Check sheet for the modelled part. Datum: model origin and axes. Units: mm. A direction names the side the tool comes from. Round coordinates to 2 decimals unless told otherwise and drop trailing zeros. Order: outer loops, then holes, each group sorted by start corner. A loop starts at its lowest first (then second) coordinate and runs counter-clockwise, first axis right, second up.
(1) Sectioned sample at A-A, the plane z = -3. Enter the section's corners in (x, y) (3 decimals).
(2) Thickness scan on probe 1 along Y at (x, z) = (38, 56.5); probe 2 along Z at (x, y) = (-33.5, 32.5) (3 decimals); probe 3 along Y at (x, z) = (22, 38.5). Record the ranges inside material, lowest first.
(3) Sectioned sample at B-B, the plane y = -28.5. Enter the section's corners in (x, z) (3 decimals).
(4) Tool access check on faces 5 (the flat face through (0, 63.5, 0)), 6 (the cylindrical face through (31.9, 16.5, 52.8)), 7 (the cylindrical face through (31.9, -16.8, 52.8)), 8 (the flat face through (47, -25.4, 42)). Record the directions out of +Z, -Z, +X, -X, +Y, -Y that give a thin tool (end or side, any length) a straight path to the whole face; none if there is none.
(5) Mould release check, pull along X, two halves, no side actions. Record for faces 1 (the flat face through (41.275, -1, 6)), 2 (the flat face through (-1, -1, -9.525)), 3 (the conical face through (84.138, 0.07, 38.115)), 4 (the cylindrical face through (44.99, -0.36, 38.95)): released by +X, released by -X, zero draft, split by the parting line, or undercut.
(6) Depth check by flat-ended pin: pin 1 (10 mm diameter, centred on y = -23, z = 45, fed in from +X); pin 2 (8 mm diameter, centred on x = 9.5, y = 44.5, fed in from +Z) (3 decimals); pin 3 (9.5 mm diameter, centred on x = 63, y = 9, fed in from +Z). Enter the tip coordinate at first touch or a pass-through.
```python
from build123d import *

# Parameters (mm, degrees)
F1_DEPTH = 63.5
F2_DEPTH = 25.4
F3_DEPTH = 7.9375
F5_R     = 6.35


with BuildPart() as f1:
    # F0 (on Front) → F1 (new body, symmetric)
    with BuildSketch(Plane.XZ):
        Polygon((41.275, -9.525), (41.275, 9.525), (22.225, 9.525), (-41.275, 9.525), (-41.275, -9.525), align=None)
    extrude(amount=F1_DEPTH, both=True)

    # F0 (on Front) → F2 (join, symmetric)
    with BuildSketch(Plane.XZ):
        with BuildLine():
            Line((22.225, 9.525), (41.275, 9.525))
            Line((41.275, 9.525), (41.275, 29.8368146303))
            ThreePointArc((41.275, 29.8368146303), (45.0938546591, 39.0563453409), (54.3133853697, 42.8752))
            Line((54.3133853697, 42.8752), (60.325, 42.8752))
            Line((60.325, 42.8752), (60.325, 61.9252))
            Line((60.325, 61.9252), (54.3133853697, 61.9252))
            ThreePointArc((54.3133853697, 61.9252), (31.6234704775, 52.5267295225), (22.225, 29.8368146303))
            Line((22.225, 29.8368146303), (22.225, 9.525))
        make_face()
        Polygon((60.325, 61.9252), (60.325, 42.8752), (85.746810308, 42.8752), (85.8338195154, 61.9252), align=None)
    extrude(amount=F2_DEPTH, both=True)

    # F0 (on Front) → F3 (join, symmetric)
    with BuildSketch(Plane.XZ):
        with BuildLine():
            Line((-41.275, 9.525), (22.225, 9.525))
            Line((22.225, 9.525), (22.225, 29.8368146303))
            ThreePointArc((22.225, 29.8368146303), (31.6234704775, 52.5267295225), (54.3133853697, 61.9252))
            add(Edge.make_bspline(
                [(-41.275, 9.525), (-39.7076308727, 40.4430106282), (10.2256173268, 62.635563314), (54.3133853697, 61.9252)],
                knots=[0, 0, 0, 0, 109.0088087157, 109.0088087157, 109.0088087157, 109.0088087157], degree=3))
        make_face()
    extrude(amount=F3_DEPTH, both=True)

    # F0 (on Front) → F4 (revolve)
    with BuildSketch(Plane.XZ):
        Polygon((85.8338195154, 61.9252), (85.746810308, 42.8752), (85.725, 38.1), (111.125, 38.1), (111.125, 66.675), (85.8555138111, 66.675), align=None)
    revolve(axis=Axis((85.7902569056, 0, 52.3875), (0.0045673648, 0, 0.9999895695)))

    # F5
    f5_edges = [f1.edges().sort_by_distance(p)[0] for p in [
        (-41.275, -63.5, 0),
        (41.275, -63.5, 0),
        (41.275, 63.5, 0),
        (-41.275, 63.5, 0),
    ]]
    fillet(f5_edges, radius=F5_R)


solid = f1.part
```
Derived:
1. outline: (-41.275, -57.15) arc R6.35 ccw to (-34.925, -63.5) - (34.925, -63.5) arc R6.35 ccw to (41.275, -57.15) - (41.275, 57.15) arc R6.35 ccw to (34.925, 63.5) - (-34.925, 63.5) arc R6.35 ccw to (-41.275, 57.15) - close
2. probe 1: y = -25.4 to 25.4
2. probe 2: z = -9.525 to 9.525
2. probe 3: y = -7.94 to 7.94
3. outline: (-41.275, -9.525) - (41.275, -9.525) - (41.275, 9.525) - (-41.275, 9.525) - close
4. face 5: +Z, -Z, +X, -X, +Y
4. face 6: +Z, -X, +Y
4. face 7: +Z, -X, -Y
4. face 8: +Z, +X, -X, -Y
5. face 1: released by +X
5. face 2: zero draft
5. face 3: undercut
5. face 4: undercut
6. pin 1: stops at x = 103.63
6. pin 2: stops at z = 9.525
6. pin 3: stops at z = 66.9
